Part model, mm, in its own coordinate system. Round coordinates to 2 decimals unless told otherwise and drop trailing zeros. Write each loop counter-clockwise with the first axis right and the second up, starting at its lowest first coordinate (ties: lowest second). Pieces come first, ordered by that corner, then holes. Notation, with made-up numbers: M 86,8 L 117,8 A27 ccw 117,25 Z; hole C -15,-2.75 d7. An arc over 180 degrees is marked long. Answer as a JSON object with one key per item and string values. Group by question number.
1. Band-saw the part on C-C, the plane x = 20. Write the cut outline in (y, z) (3 decimals).
2. Drill centre lines: line 1 (Y direction, x = -22, z = 0.9); line 2 (X direction, y = 21, z = 1.5); line 3 (X direction, y = 11, z = 2.2). Where is each one in solid material? Low to high. Write a range as from..to.
3. Band-saw the part on A-A, the plane x = 0. Write the cut outline in (y, z) (3 decimals).
4. Drop flat-ended pins along their axis: pin 1 (1.5 mm diameter, centred on y = -7.5, z = 0.5, fed in from +X); pin 2 (6.5 mm diameter, centred on x = -7.43, y = 27.74, fed in from +Z) (3 decimals); pin 3 (3 mm diameter, centred on x = 0, y = 28.72, fed in from +Z); pin 4 (1 mm diameter, centred on x = -10, z = 2, fed in from +Y). Give the stop position or say it passes through.
5. Band-saw the part on D-D, the plane y = -28.72. Write the cut outline in (x, z) (3 decimals), plus the area to 3 significant figures.
from build123d import *

# Parameters (mm, degrees)
SKETCH1_R           = 33.8
SKETCH1_R_2         = 2.54
SKETCH1_R_3         = 2.05
SKETCH1_R_4         = 0.75
SKETCH1_W           = 3.048
SKETCH1_H           = 19.05
SKETCH1_W_2         = 19.05
SKETCH1_H_2         = 3.048
BOSS_EXTRUDE1_DEPTH = 3.175


with BuildPart() as part:
    # Sketch1 → Boss-Extrude1 (new body)
    with BuildSketch(Plane.XY):
        Circle(SKETCH1_R)
        with Locations((14.36, 24.872249597)):
            Circle(SKETCH1_R_2, mode=Mode.SUBTRACT)
        with Locations((20.308106756, 20.308106756)):
            Circle(SKETCH1_R_2, mode=Mode.SUBTRACT)
        with Locations((24.872249597, 14.36)):
            Circle(SKETCH1_R_2, mode=Mode.SUBTRACT)
        with Locations((27.741389731, 7.433282975)):
            Circle(SKETCH1_R_2, mode=Mode.SUBTRACT)
        with Locations((28.72, 0)):
            Circle(SKETCH1_R_2, mode=Mode.SUBTRACT)
        with Locations((27.741389731, -7.433282975)):
            Circle(SKETCH1_R_2, mode=Mode.SUBTRACT)
        with Locations((24.872249597, -14.36)):
            Circle(SKETCH1_R_2, mode=Mode.SUBTRACT)
        with Locations((20.308106756, -20.308106756)):
            Circle(SKETCH1_R_2, mode=Mode.SUBTRACT)
        with Locations((14.36, -24.872249597)):
            Circle(SKETCH1_R_2, mode=Mode.SUBTRACT)
        with Locations((7.433282975, -27.741389731)):
            Circle(SKETCH1_R_2, mode=Mode.SUBTRACT)
        with Locations((0, -28.72)):
            Circle(SKETCH1_R_2, mode=Mode.SUBTRACT)
        with Locations((-7.433282975, -27.741389731)):
            Circle(SKETCH1_R_2, mode=Mode.SUBTRACT)
        with Locations((-14.36, -24.872249597)):
            Circle(SKETCH1_R_2, mode=Mode.SUBTRACT)
        with Locations((-20.308106756, -20.308106756)):
            Circle(SKETCH1_R_2, mode=Mode.SUBTRACT)
        with Locations((-24.872249597, -14.36)):
            Circle(SKETCH1_R_2, mode=Mode.SUBTRACT)
        with Locations((-27.741389731, -7.433282975)):
            Circle(SKETCH1_R_2, mode=Mode.SUBTRACT)
        with Locations((-28.72, 0)):
            Circle(SKETCH1_R_2, mode=Mode.SUBTRACT)
        with Locations((-27.741389731, 7.433282975)):
            Circle(SKETCH1_R_2, mode=Mode.SUBTRACT)
        with Locations((-24.872249597, 14.36)):
            Circle(SKETCH1_R_2, mode=Mode.SUBTRACT)
        with Locations((-20.308106756, 20.308106756)):
            Circle(SKETCH1_R_2, mode=Mode.SUBTRACT)
        with Locations((-14.36, 24.872249597)):
            Circle(SKETCH1_R_2, mode=Mode.SUBTRACT)
        with Locations((-7.433282975, 27.741389731)):
            Circle(SKETCH1_R_2, mode=Mode.SUBTRACT)
        with Locations((0, 28.72)):
            Circle(SKETCH1_R_2, mode=Mode.SUBTRACT)
        with Locations((7.433282975, 27.741389731)):
            Circle(SKETCH1_R_2, mode=Mode.SUBTRACT)
        Circle(SKETCH1_R_3, mode=Mode.SUBTRACT)
        with Locations((11.561195872, 11.561195872)):
            Circle(SKETCH1_R_4, mode=Mode.SUBTRACT)
        with Locations((9.439875529, 9.439875529)):
            Circle(SKETCH1_R_4, mode=Mode.SUBTRACT)
        with Locations((7.318555185, 7.318555185)):
            Circle(SKETCH1_R_4, mode=Mode.SUBTRACT)
        with Locations((5.197234842, 5.197234842)):
            Circle(SKETCH1_R_4, mode=Mode.SUBTRACT)
        with Locations((11.561195872, -11.561195872)):
            Circle(SKETCH1_R_4, mode=Mode.SUBTRACT)
        with Locations((9.439875529, -9.439875529)):
            Circle(SKETCH1_R_4, mode=Mode.SUBTRACT)
        with Locations((7.318555185, -7.318555185)):
            Circle(SKETCH1_R_4, mode=Mode.SUBTRACT)
        with Locations((5.197234842, -5.197234842)):
            Circle(SKETCH1_R_4, mode=Mode.SUBTRACT)
        with Locations((-11.561195872, -11.561195872)):
            Circle(SKETCH1_R_4, mode=Mode.SUBTRACT)
        with Locations((-9.439875529, -9.439875529)):
            Circle(SKETCH1_R_4, mode=Mode.SUBTRACT)
        with Locations((-7.318555185, -7.318555185)):
            Circle(SKETCH1_R_4, mode=Mode.SUBTRACT)
        with Locations((-5.197234842, -5.197234842)):
            Circle(SKETCH1_R_4, mode=Mode.SUBTRACT)
        with Locations((-11.561195872, 11.561195872)):
            Circle(SKETCH1_R_4, mode=Mode.SUBTRACT)
        with Locations((-9.439875529, 9.439875529)):
            Circle(SKETCH1_R_4, mode=Mode.SUBTRACT)
        with Locations((-7.318555185, 7.318555185)):
            Circle(SKETCH1_R_4, mode=Mode.SUBTRACT)
        with Locations((-5.197234842, 5.197234842)):
            Circle(SKETCH1_R_4, mode=Mode.SUBTRACT)
        with Locations((0, 14.115)):
            Rectangle(SKETCH1_W, SKETCH1_H, mode=Mode.SUBTRACT)
        with Locations((14.115, 0)):
            Rectangle(SKETCH1_W_2, SKETCH1_H_2, mode=Mode.SUBTRACT)
        with Locations((0, -14.115)):
            Rectangle(SKETCH1_W, SKETCH1_H, mode=Mode.SUBTRACT)
        with Locations((-14.115, 0)):
            Rectangle(SKETCH1_W_2, SKETCH1_H_2, mode=Mode.SUBTRACT)
    extrude(amount=BOSS_EXTRUDE1_DEPTH)


solid = part.part
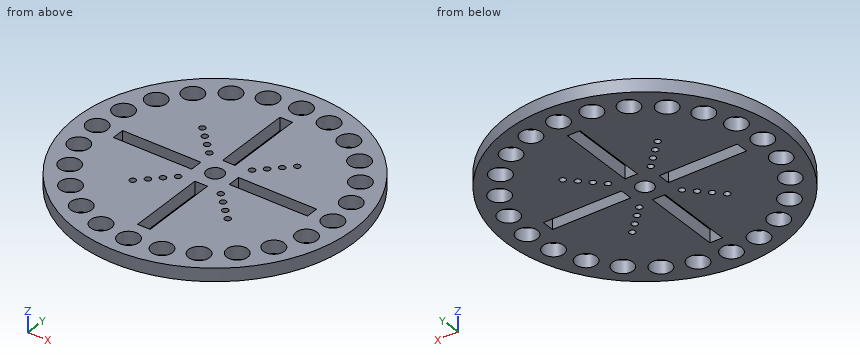
Worked answers:
{
 "1": {"outline": "M -27.248,0 L -22.829,0 L -22.829,3.175 L -27.248,3.175 Z; M -17.787,0 L -1.524,0 L -1.524,3.175 L -17.787,3.175 Z; M 1.524,0 L 17.787,0 L 17.787,3.175 L 1.524,3.175 Z; M 22.829,0 L 27.248,0 L 27.248,3.175 L 22.829,3.175 Z"},
 "2": {"line 1": "y = -25.66..-22.2, -18.41..-1.52, 1.52..18.41, 22.2..25.66", "line 2": "x = -26.48..-22.75, -17.86..-1.52, 1.52..17.86, 22.75..26.48", "line 3": "x = -31.96..-12.06, -11.06..-1.52, 1.52..11.06, 12.06..31.96"},
 "3": {"outline": "M -33.8,0 L -31.26,0 L -31.26,3.175 L -33.8,3.175 Z; M -26.18,0 L -23.64,0 L -23.64,3.175 L -26.18,3.175 Z; M -4.59,0 L -2.05,0 L -2.05,3.175 L -4.59,3.175 Z; M 2.05,0 L 4.59,0 L 4.59,3.175 L 2.05,3.175 Z; M 23.64,0 L 26.18,0 L 26.18,3.175 L 23.64,3.175 Z; M 31.26,0 L 33.8,0 L 33.8,3.175 L 31.26,3.175 Z"},
 "4": {"pin 1": "stops at x = 33.12", "pin 2": "stops at z = 3.175", "pin 3": "passes through", "pin 4": "stops at y = 32.44"},
 "5": {"outline": "M -17.821,0 L -9.777,0 L -9.777,3.175 L -17.821,3.175 Z; M -5.089,0 L -2.54,0 L -2.54,3.175 L -5.089,3.175 Z; M 2.54,0 L 5.089,0 L 5.089,3.175 L 2.54,3.175 Z; M 9.777,0 L 17.821,0 L 17.821,3.175 L 9.777,3.175 Z", "area": "67.3 mm^2"}
}
